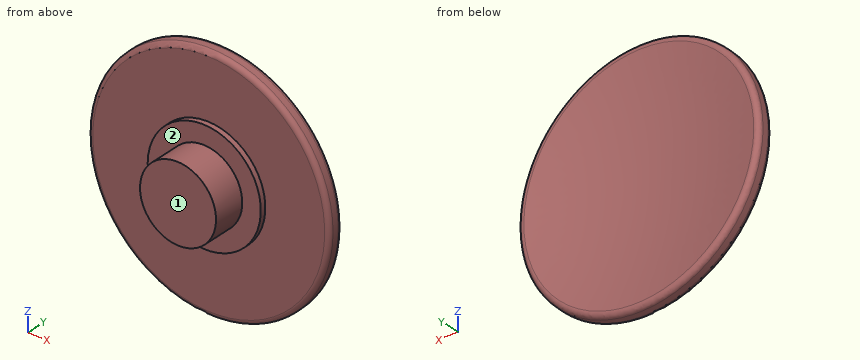
```python
from build123d import *

# Parameters (mm, degrees)
F2_R = 0.5


with BuildPart() as f1:
    # F0 (on Top) → F1 (revolve)
    with BuildSketch(Plane.XY):
        with BuildLine():
            ThreePointArc((0, 14.924920715), (-6.5431261642, 15.3011606257), (-13, 16.424920715))
            Line((-13, 16.424920715), (-13, 14.624920715))
            Line((-13, 14.624920715), (-6.1, 14.624920715))
            Line((-6.1, 14.624920715), (-6.1, 14.024920715))
            Line((-6.1, 14.024920715), (-4.1, 14.024920715))
            Line((-4.1, 14.024920715), (-4.1, 10.524920715))
            Line((-4.1, 10.524920715), (0, 10.524920715))
            Line((0, 10.524920715), (0, 14.924920715))
        make_face()
    revolve(axis=Axis((0, 12.724920715, 0), (0, 1, 0)))

    # F2
    f2_edges = [f1.edges().sort_by_distance(p)[0] for p in [
        (13, 14.624921, 0),
        (13, 16.424921, 0),
    ]]
    fillet(f2_edges, radius=F2_R)


solid = f1.part
```
The listing builds one solid part. Answer for the finished solid, in the listing's coordinates (mm). Face numbers are marked on the shaded views. A direction names the side the tool comes from. Round coordinates to 2 decimals unless told otherwise and drop trailing zeros. Write each loop counter-clockwise with the first axis right and the second up, starting at its lowest first coordinate (ties: lowest second). Pieces come first, ordered by that corner, then holes. Notation, with made-up numbers: (17.25, 83.5) -> (34.25, 83.5) arc R15 cw to (34.25, 99.5) -> close; hole circle Ø6 at (88, 45). An arc over 180 degrees is marked (long way). Write item = value, one per line.
1) Section A-A on y = 13.25 is taken. Write down the section's boundary in (x, z), plus the area to 3 significant figures.
Check values:
outline = circle Ø8.2 at (0, 0)
area = 52.8 mm²
2) Given pin 1 (1.5 mm diameter, centred on y = 14.5, z = -1.5, fed in from -X); pin 2 (1 mm diameter, centred on y = 15, z = -2.5, fed in from -X); pin 3 (3 mm diameter, centred on y = 12, z = -6.5, fed in from +X), each flat-ended and moving along its own axis, determine where each tip first touches the part or whether it passes through.
Check values:
pin_1 = -12.96
pin_2 = -12.84
pin_3 = through
3) Straight lines are drawn through the part: line 1 along Y through (x, z) = (-0.25, 0.75); line 2 along Z through (x, y) = (0.25, 14.1); line 3 along X through (y, z) = (14.85, -5.5). For each, find the intervals that lie inside material, in ascending order. Write a range as [from, to].
Check values:
line_1 = [10.52, 14.93]
line_2 = [-6.09, 6.09]
line_3 = [-11.69, 11.69]
4) Which of the six approach directions +Z, -Z, +X, -X, +Y, -Y give full straight-line access (tool end or side, diameter ignored) to the marked faces 1 and 2?
Check values:
face_1 = +Z, -Z, +X, -X, -Y
face_2 = -Y
